Here's the drawing with two shaded views (mm, measured from the low corner). I have some questions. A direction names the side the tool comes from. Give positions to 0.01 mm unless a question says otherwise; leave off trailing zeros. Loops run counter-clockwise (first coordinate to the right, second up) from the corner with the lowest first, then second, coordinate; pieces in that order, holes last. Notation, with made-up numbers: M 65.5,39.5 L 84.5,39.5 A21 ccw 84.5,68.5 Z; hole C 72.25,59.25 d1. An arc over 180 degrees is marked long. Write item = value, one per line. Start each with the question number.
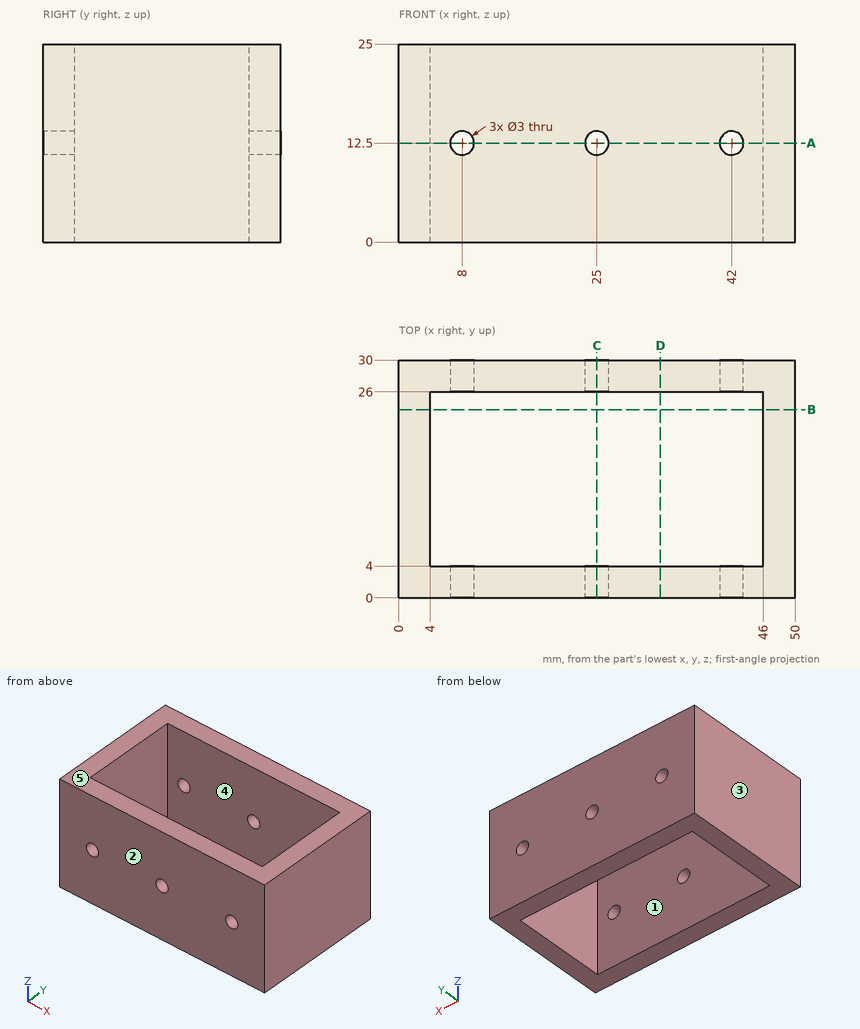
Q1. If I drill on line 1 along Z through (x, y) = (8, 1.5); line 2 along Y through (x, z) = (40, 22); line 3 along X through (y, z) = (22.25, 13.25), over which ranges is the centre line in solid material (lowest first)?
Q2. If we section it at A-A, the plane z = 12.5: State how many separate pieces and enclosed holes the cut face has, then the cut area to 3 significant figures.
Q3. If we section it at D-D, the plane x = 33: List the corners of the cut face in (y, z) for me, then the cut area to 3 significant figures.
Q4. If we section it at B-B, the plane y = 23.75: List the corners of the cut face in (x, z) for me, then the cut area to 3 significant figures.
Q5. On a 3-axis mill with a long thin cutter (end or side, diameter ignored), from which of +Z, -Z, +X, -X, +Y, -Y can I reach the whole of each face in a straight line? I mean the marked faces 4 and 5. Say none if no direction works.
Q6. We'd pull the mould along X, two halves only. Please class the marked faces 1, 2 and 3: pulls with the +X half, pulls with the -X half, needs draft (parallel to the pull), parting line crosses it, or undercut.
Q7. If we section it at C-C, the plane x = 25: List the corners of the cut face in (y, z) for me, then the cut area to 3 significant figures.
Q8. Will this pin go through, and if not, where does the flat tip stop? pin 1 (2 mm diameter, centred on x = 19, y = 24, fed in from +Z).
Resolved:
q1.line_1 = 0 to 11, 14 to 25
q1.line_2 = 0 to 4, 26 to 30
q1.line_3 = 0 to 4, 46 to 50
q2.separate_pieces = 6
q2.enclosed_holes = 0
q2.area = 504 mm²
q3.outline = M 0,0 L 4,0 L 4,25 L 0,25 Z; M 26,0 L 30,0 L 30,25 L 26,25 Z
q3.area = 200 mm²
q4.outline = M 0,0 L 4,0 L 4,25 L 0,25 Z; M 46,0 L 50,0 L 50,25 L 46,25 Z
q4.area = 200 mm²
q5.face_4 = +Z, -Z
q5.face_5 = +Z, +X, -X, +Y, -Y
q6.face_1 = undercut
q6.face_2 = needs draft
q6.face_3 = pulls with the -X half
q7.outline = M 0,0 L 4,0 L 4,11 L 0,11 Z; M 0,14 L 4,14 L 4,25 L 0,25 Z; M 26,0 L 30,0 L 30,11 L 26,11 Z; M 26,14 L 30,14 L 30,25 L 26,25 Z
q7.area = 176 mm²
q8.pin_1 = through
